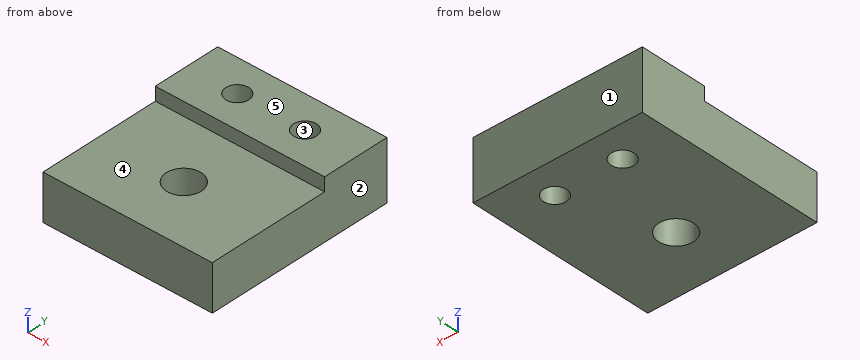
```python
from build123d import *

# Parameters (mm, degrees)
SKETCH1_W           = 31.75
SKETCH1_H           = 12.7
SKETCH1_R           = 2.15265
BOSS_EXTRUDE1_DEPTH = 11.0998
SKETCH1_6_W         = 31.75
SKETCH1_6_H         = 22.86
SKETCH1_6_R         = 3.2639
BOSS_EXTRUDE2_DEPTH = 8.5598


with BuildPart() as part:
    # Sketch1 → Boss-Extrude1 (new body)
    with BuildSketch(Plane.XY):
        with Locations((15.875, 29.21)):
            Rectangle(SKETCH1_W, SKETCH1_H)
        with Locations((9.525, 29.21)):
            Circle(SKETCH1_R, mode=Mode.SUBTRACT)
        with Locations((22.225, 29.21)):
            Circle(SKETCH1_R, mode=Mode.SUBTRACT)
    extrude(amount=BOSS_EXTRUDE1_DEPTH)

    # Sketch1<6> → Boss-Extrude2 (add)
    with BuildSketch(Plane.XY):
        with Locations((15.875, 11.43)):
            Rectangle(SKETCH1_6_W, SKETCH1_6_H)
        with Locations((15.875, 11.43)):
            Circle(SKETCH1_6_R, mode=Mode.SUBTRACT)
    extrude(amount=BOSS_EXTRUDE2_DEPTH)


solid = part.part
```
The model under review builds one solid part; all positions refer to its coordinate system, in mm. Face numbers are marked on the shaded views. A direction names the side the tool comes from. Coordinates: 2 decimals unless noted, no trailing zeros. Write each loop counter-clockwise with the first axis right and the second up, starting at its lowest first coordinate (ties: lowest second). Pieces come first, ordered by that corner, then holes. Notation, with made-up numbers: (-9.75, 78.25) - (43.25, 78.25) arc R33 cw to (43.25, 107.25) - close; hole circle Ø9 at (25, 84). An arc over 180 degrees is marked (long way). Write item = value, one per line.
(1) Machinability: for the marked faces 4 and 5, which of the approach directions +Z, -Z, +X, -X, +Y, -Y give a long, thin tool a straight path to every point of the face, cutting with its end or side? Answer none if there is none.
Result sheet:
face_4 = +Z, +X, -X, -Y
face_5 = +Z, +X, -X, +Y, -Y
(2) Consider section B-B, the plane z = 7.25. Give the boundary of the cut face in (x, y) (3 decimals), then the cut area to 3 significant figures.
Result sheet:
outline = (0, 0) - (31.75, 0) - (31.75, 35.56) - (0, 35.56) - close; hole circle Ø4.305 at (9.525, 29.21); hole circle Ø6.528 at (15.875, 11.43); hole circle Ø4.305 at (22.225, 29.21)
area = 1,070 mm^2
(3) For P1, Ø2.5, axis at x = 22.225, y = 29.21, coming from the -Z side; P2, Ø2, axis at x = 18, z = 10, coming from the -Y side, all flat-tipped, find the tip position at first contact; note any pin that passes through.
Result sheet:
P1 = through
P2 = 22.86
(4) Consider section D-D, the plane y = 11.43. Give the boundary of the cut face in (x, z), then the cut area to 3 significant figures.
Result sheet:
outline = (0, 0) - (12.61, 0) - (12.61, 8.56) - (0, 8.56) - close; (19.14, 0) - (31.75, 0) - (31.75, 8.56) - (19.14, 8.56) - close
area = 216 mm^2
(5) For line 1 (Y direction, x = 9, z = 0.5); line 2 (Z direction, x = 30, y = 19); line 3 (X direction, y = 13, z = 2.75), list the stretches that pass through material, from the lowest coordinate up. Write a range as [from, to].
Result sheet:
line_1 = [0, 27.12], [31.3, 35.56]
line_2 = [0, 8.56]
line_3 = [0, 13.01], [18.74, 31.75]
(6) Mouldability with a two-part tool opening along Y and no side actions: class the marked faces 1, 2 and 3 as pulls with the +Y half, pulls with the -Y half, needs draft (parallel to the pull), parting line crosses it, or undercut.
Result sheet:
face_1 = pulls with the +Y half
face_2 = needs draft
face_3 = undercut
(7) Consider section A-A, the plane y = 29.21. Give the boundary of the cut face in (x, z).
Result sheet:
outline = (0, 0) - (7.37, 0) - (7.37, 11.1) - (0, 11.1) - close; (11.68, 0) - (20.07, 0) - (20.07, 11.1) - (11.68, 11.1) - close; (24.38, 0) - (31.75, 0) - (31.75, 11.1) - (24.38, 11.1) - close
(8) Consider section C-C, the plane x = 22.5. Give the boundary of the cut face in (y, z).
Result sheet:
outline = (0, 0) - (27.07, 0) - (27.07, 11.1) - (22.86, 11.1) - (22.86, 8.56) - (0, 8.56) - close; (31.35, 0) - (35.56, 0) - (35.56, 11.1) - (31.35, 11.1) - close
